Geometry: final body of the model. Coordinates: model frame, mm. Face numbers are marked on the shaded views. A direction names the side the tool comes from. Round coordinates to 2 decimals unless told otherwise and drop trailing zeros. Loops run counter-clockwise (first coordinate to the right, second up) from the corner with the lowest first, then second, coordinate; pieces in that order, holes last. Notation, with made-up numbers: (66.25, 45) - (122.25, 45) arc R31 cw to (122.25, 79) - close; hole circle Ø9 at (85, 52.25). An arc over 180 degrees is marked (long way). Write item = value, one per line. Start each with the question number.
Item 1: First-contact query: pin 1 (1 mm diameter, centred on x = -12, z = 103.5, fed in from -Y); pin 2 (5 mm diameter, centred on y = -1, z = 38, fed in from +X); pin 3 (1 mm diameter, centred on y = -5, z = 25, fed in from -X); pin 4 (11 mm diameter, centred on y = 0, z = 84, fed in from +X). Flat tips, straight axial feed; report the tip coordinate or a pass-through.
Item 2: Line query: line 1 (Z direction, x = 3, y = -17); line 2 (Z direction, x = 1.5, y = -4); line 3 (X direction, y = 0, z = 28). Output: solid intervals per line, ascending. Write a range as from..to.
Item 3: Draft query along X for the marked faces 1 and 2. Return one class per face: pulls with the +X half, pulls with the -X half, needs draft (parallel to the pull), parting line crosses it, or undercut.
Item 4: Access query for the marked faces 3, 4 and 5. Directions: +Z, -Z, +X, -X, +Y, -Y. A direction counts if a zero-diameter tool reaches every point of the face in a straight line with its end or side. Return the directions, or none.
Item 5: Section A-A (z = 31.5). Return loops of the section in (x, y), plus the area to 3 significant figures.
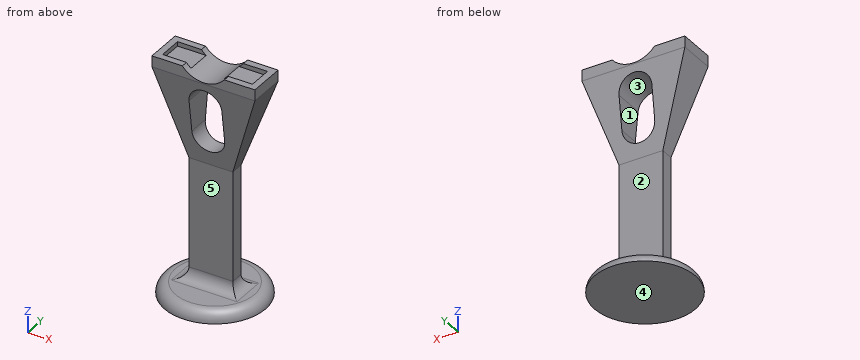
from build123d import *

# Parameters (mm, degrees)
F1_W       = 41
F1_H       = 11
F2_DEPTH   = 3
F1_W_2     = 47
F1_H_2     = 17
F3_DEPTH   = 5
F5_DEPTH   = 17.001
F6_R       = 23
F7_DEPTH   = 5
F8_W       = 20
F8_H       = 6
F9_DEPTH   = 55
F9_FACE_W  = 20
F9_FACE_H  = 6
F3_FACE1_W = 47
F3_FACE1_H = 17
F12_DEPTH  = 25
F13_R      = 4.99999


# Not quite as in the source:
# - a fillet or chamfer is up to 0.001 mm smaller than in the source, because OpenCascade refuses the exact size


with BuildPart() as f2:
    # F1 (on offset) → F2 (new body)
    with BuildSketch(Plane.XY.offset(100)):
        Rectangle(F1_W, F1_H)
    extrude(amount=F2_DEPTH)

    # F1 (on offset) → F3 (join)
    with BuildSketch(Plane.XY.offset(100)):
        Rectangle(F1_W_2, F1_H_2)
        Rectangle(F1_W, F1_H, mode=Mode.SUBTRACT)
    extrude(amount=F3_DEPTH)

    # F4 (on face) → F5 (cut, through all)
    with BuildSketch(Plane.XZ.offset(8.5)):
        with BuildLine():
            Line((9.6046863561, 105), (-9.6046863561, 105))
            ThreePointArc((-9.6046863561, 105), (0, 100.5), (9.6046863561, 105))
        make_face()
    extrude(amount=-F5_DEPTH, mode=Mode.SUBTRACT)



with BuildPart() as f7:
    # F6 (on Top) → F7 (new body)
    with BuildSketch(Plane.XY):
        Circle(F6_R)
    extrude(amount=F7_DEPTH)

    # F8 (on face) → F9 (join)
    with BuildSketch(Plane.XY.offset(5)):
        Rectangle(F8_W, F8_H)
    extrude(amount=F9_DEPTH)


with BuildPart() as f2_1:
    add(f2.part)

    add(f7.part)  # F10 merges F7
    # F9_face (on face) → F10 section 0
    with BuildSketch(Plane.XY.offset(60)):
        Rectangle(F9_FACE_W, F9_FACE_H)
    # F3_face1 (on face) → F10 section 1
    with BuildSketch(Plane(origin=(0, 0, 100), x_dir=(1, 0, 0), z_dir=(0, 0, -1))):
        Rectangle(F3_FACE1_W, F3_FACE1_H)
    loft()

    # F11 (on Front) → F12 (cut, symmetric)
    with BuildSketch(Plane.XZ):
        with BuildLine():
            ThreePointArc((7.5, 89), (0, 96.5), (-7.5, 89))
            Line((-7.5, 89), (-7.5, 74))
            ThreePointArc((-7.5, 74), (0, 66.5), (7.5, 74))
            Line((7.5, 74), (7.5, 89))
        make_face()
    extrude(amount=F12_DEPTH, both=True, mode=Mode.SUBTRACT)

    # F13 (radius 5 in the source; OpenCascade refuses exactly that, so slightly less here)
    f13_edges = [f2_1.edges().sort_by_distance(p)[0] for p in [
        (0, -3, 5),
        (-10, 0, 5),
        (0, 3, 5),
        (10, 0, 5),
        (-23, 0, 5),
    ]]
    fillet(f13_edges, radius=F13_R)


solid = f2_1.part
Taken from the geometry:
q1.pin_1 = -8.5
q1.pin_2 = 10
q1.pin_3 = through
q1.pin_4 = 19.96
q2.line_1 = 0..5
q2.line_2 = 0..7, 96.35..100.59
q2.line_3 = -10..10
q3.face_1 = undercut
q3.face_2 = needs draft
q4.face_3 = +Y, -Y
q4.face_4 = -Z, +X, -X, +Y, -Y
q4.face_5 = +X, -X, -Y
q5.outline = (-10, -3) - (10, -3) - (10, 3) - (-10, 3) - close
q5.area = 120 mm^2
